Geometry check sheet. Reference: the model listing, model coordinates, mm. A direction names the side the tool comes from. Give positions to 0.01 mm unless a question says otherwise; leave off trailing zeros. Order: outer loops, then holes, each group sorted by start corner. A loop starts at its lowest first (then second) coordinate and runs counter-clockwise, first axis right, second up. Notation, with made-up numbers: M 19,-32.75 L 43,-32.75 A29 cw 43,5.25 Z; hole C 61.5,68.25 d7. An arc over 180 degrees is marked long. Answer as a JSON object with one key per item and string values. Group by question number.
from build123d import *

# Parameters (mm, degrees)
F1_DEPTH = 40
F2_W     = 14.6631337702
F2_H     = 28.3150114119
F3_DEPTH = 2
F5_DEPTH = 1
F6_R     = 3
F6_R_2   = 4
F7_DEPTH = 1


# Not quite as in the source:
# - a pattern or mirror of a feature is missing from the dataset's text; its kind, count and spacing are read off the source's solid


with BuildPart() as f1:
    # F0 (on Right) → F1 (new body, symmetric)
    with BuildSketch(Plane.YZ):
        with BuildLine():
            Line((74.1590947979, 0), (74.1590947979, 80))
            Line((74.1590947979, 80), (4.1590947979, 80))
            Line((4.1590947979, 80), (-5.8409052021, 30))
            Line((-5.8409052021, 30), (-45.8409052021, 30))
            Line((-45.8409052021, 30), (-45.8409052021, 0))
            Line((-45.8409052021, 0), (-22.3770336471, 0))
            ThreePointArc((-22.3770336471, 0), (-9.8770336471, 12.5), (2.6229663529, 0))
            Line((2.6229663529, 0), (30.7202589484, 0))
            ThreePointArc((30.7202589484, 0), (43.2202589484, 12.5), (55.7202589484, 0))
            Line((55.7202589484, 0), (74.1590947979, 0))
        make_face()
        with BuildLine():
            ThreePointArc((30.7202589484, 0), (43.2202589484, -12.5), (55.7202589484, 0))
            Line((55.7202589484, 0), (30.7202589484, 0))
        make_face()
        with BuildLine():
            Line((30.7202589484, 0), (55.7202589484, 0))
            ThreePointArc((55.7202589484, 0), (43.2202589484, 12.5), (30.7202589484, 0))
        make_face()
        with BuildLine():
            ThreePointArc((-22.3770336471, 0), (-9.8770336471, -12.5), (2.6229663529, 0))
            Line((2.6229663529, 0), (-22.3770336471, 0))
        make_face()
        with BuildLine():
            Line((-22.3770336471, 0), (2.6229663529, 0))
            ThreePointArc((2.6229663529, 0), (-9.8770336471, 12.5), (-22.3770336471, 0))
        make_face()
    extrude(amount=F1_DEPTH, both=True)

    # F2 (on face) → F3 (cut)
    with BuildSketch(Plane(origin=(-40, 0, 0), x_dir=(0, -1, 0), z_dir=(-1, 0, 0))):
        Polygon((-13.9850862324, 40.0354526937), (-25.6144665182, 69.0246298909), (-39.0978083014, 68.3504641056), (-39.0978083014, 40.2039922774), align=None)
        with Locations((-59.0700041503, 54.1929583997)):
            Rectangle(F2_W, F2_H)
    f3 = extrude(amount=-F3_DEPTH, mode=Mode.SUBTRACT)

    # F3_copies: F3 across plane
    add(f3.mirror(Plane(origin=(0, 0, 0), x_dir=(0, 0, 1), z_dir=(1, 0, 0))), mode=Mode.SUBTRACT)

    # F4 (on face) → F5 (cut, symmetric)
    with BuildSketch(Plane(origin=(0, -11.3854857713, 2.2770971543), x_dir=(1, 0, 0), z_dir=(0, -0.9805806757, 0.1961161351))):
        Polygon((35.1756438613, 74.5268389583), (-35.977371037, 74.3224471807), (-35.977371037, 34.0555720031), (35.1756438613, 34.0555720031), align=None)
    extrude(amount=F5_DEPTH, both=True, mode=Mode.SUBTRACT)

    # F6 (on face) → F7 (cut, symmetric)
    with BuildSketch(Plane.XZ.offset(45.8409052021)):
        with Locations((-34, 15)):
            Circle(F6_R)
        with Locations((-24, 15)):
            Circle(F6_R_2)
        with Locations((24, 15)):
            Circle(F6_R_2)
        with Locations((34, 15)):
            Circle(F6_R)
    extrude(amount=F7_DEPTH, both=True, mode=Mode.SUBTRACT)


solid = f1.part
1. Access from +Z, -Z, +X, -X, +Y, -Y to the whole of each face (thin tool, end or side, straight path). Record for faces 4 (the flat face through (-24, -44.841, 15)), 5 (the flat face through (-38, 59, 54)), 6 (the flat face through (38, 30, 55)), 7 (the flat face through (1, -34, 0)), 8 (the flat face through (1, 65, 0)).
2. Release check for a two-part mould opening along Y. For faces 1 (the flat face through (1, 40, 80)), 2 (the flat face through (1, 74.159, 39)), 3 (the flat face through (1, 16, 0)) record: released by +Y, released by -Y, zero draft, split by the parting line, or undercut.
3. Thickness scan on line 1 along Z through (x, y) = (-24, -45.05); line 2 along Y through (x, z) = (-4, 54); line 3 along Z through (x, y) = (17.5, 43). Record the ranges inside material, lowest first. Write a range as [from, to].
4. Cross-section at B-B (x = -25). Record the cut outline in (y, z).
5. Cross-section at C-C (y = 27.5). Record the cut outline in (x, z).
6. Cross-section at A-A (z = -6). Record the cut outline in (x, y), and give its area (3 significant figures).
7. Depth check by flat-ended pin: pin 1 (1 mm diameter, centred on x = -24, y = -33.5, fed in from +Z); pin 2 (5 mm diameter, centred on x = -15, z = 39, fed in from -Y); pin 3 (1 mm diameter, centred on x = 39.5, y = 62.5, fed in from -Z). Enter the tip coordinate at first touch or a pass-through.
8. Cross-section at D-D (z = 65). Record the cut outline in (x, y).
Report:
{
 "1": {"face 4": "-Y", "face 5": "-X", "face 6": "+X", "face 7": "-Z, +X, -X, -Y", "face 8": "-Z, +X, -X, +Y"},
 "2": {"face 1": "zero draft", "face 2": "released by +Y", "face 3": "undercut"},
 "3": {"line 1": "z = [0, 11], [19, 30]", "line 2": "y = [-0.02, 74.16]", "line 3": "z = [-12.5, 80]"},
 "4": {"outline": "M -45.84,0 L -22.38,0 A12.5 ccw 2.62,0 L 30.72,0 A12.5 ccw 55.72,0 L 74.16,0 L 74.16,80 L 4.16,80 L 3.2,75.19 L 4.18,74.99 L -3.73,35.48 L -4.71,35.67 L -5.84,30 L -45.84,30 L -45.84,18.87 L -44.84,18.87 L -44.84,11.13 L -45.84,11.13 Z"},
 "5": {"outline": "M -40,0 L 40,0 L 40,40.13 L 38,40.13 L 38,68.93 L 40,68.93 L 40,80 L -40,80 L -40,68.93 L -38,68.93 L -38,40.13 L -40,40.13 Z"},
 "6": {"outline": "M -40,-20.84 L 40,-20.84 L 40,1.09 L -40,1.09 Z; M -40,32.25 L 40,32.25 L 40,54.19 L -40,54.19 Z", "area": "3,510 mm2"},
 "7": {"pin 1": "stops at z = 30", "pin 2": "stops at y = -3.52", "pin 3": "stops at z = 0"},
 "8": {"outline": "M -40,1.16 L -35.98,1.16 L -35.98,2.18 L 35.18,2.18 L 35.18,1.16 L 40,1.16 L 40,24 L 38,24 L 38,39.1 L 40,39.1 L 40,51.74 L 38,51.74 L 38,66.4 L 40,66.4 L 40,74.16 L -40,74.16 L -40,66.4 L -38,66.4 L -38,51.74 L -40,51.74 L -40,39.1 L -38,39.1 L -38,24 L -40,24 Z"}
}
